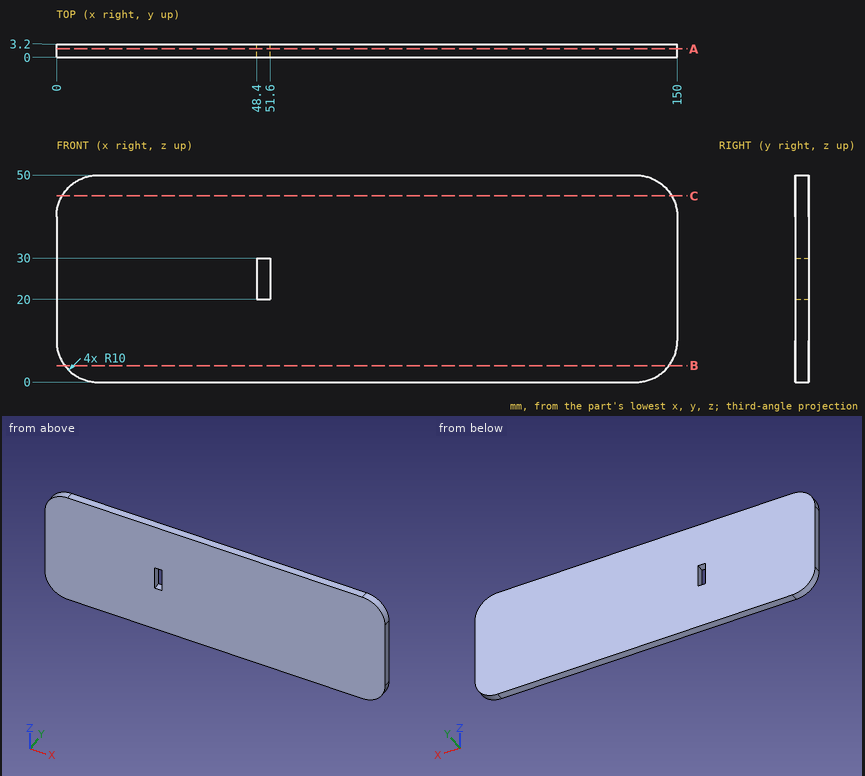
Drawing for the job (mm, zero at the part's lowest x, y, z). Round coordinates to 2 decimals unless told otherwise and drop trailing zeros. Order: outer loops, then holes, each group sorted by start corner. A loop starts at its lowest first (then second) coordinate and runs counter-clockwise, first axis right, second up. Notation, with made-up numbers: (74.25, 85.5) -> (85.25, 85.5) arc R11 cw to (85.25, 90.5) -> close; hole circle Ø3 at (-5, 60). An arc over 180 degrees is marked (long way). Write item = value, one per line. Start each with the question number.
(1) Cut at A-A, the plane y = 2. List the corners of the cut face in (x, z), then the cut area to 3 significant figures.
(2) Cut at C-C, the plane z = 45. List the corners of the cut face in (x, y), then the cut area to 3 significant figures.
(3) Probe line 1 (X direction, y = 2.75, z = 25.5); line 2 (X direction, y = 0.2, z = 42.5); line 3 (X direction, y = 2.45, z = 45.5). List the from-to ranges inside material, lowest first. Write a range as [from, to].
(4) Cut at B-B, the plane z = 4. List the corners of the cut face in (x, y).
Model answer:
q1.outline = (0, 10) arc R10 ccw to (10, 0) -> (140, 0) arc R10 ccw to (150, 10) -> (150, 40) arc R10 ccw to (140, 50) -> (10, 50) arc R10 ccw to (0, 40) -> close; hole (48.4, 20) -> (51.6, 20) -> (51.6, 30) -> (48.4, 30) -> close
q1.area = 7,380 mm2
q2.outline = (1.34, 0) -> (148.66, 0) -> (148.66, 3.2) -> (1.34, 3.2) -> close
q2.area = 471 mm2
q3.line_1 = [0, 48.4], [51.6, 150]
q3.line_2 = [0.32, 149.68]
q3.line_3 = [1.65, 148.35]
q4.outline = (2, 0) -> (148, 0) -> (148, 3.2) -> (2, 3.2) -> close
